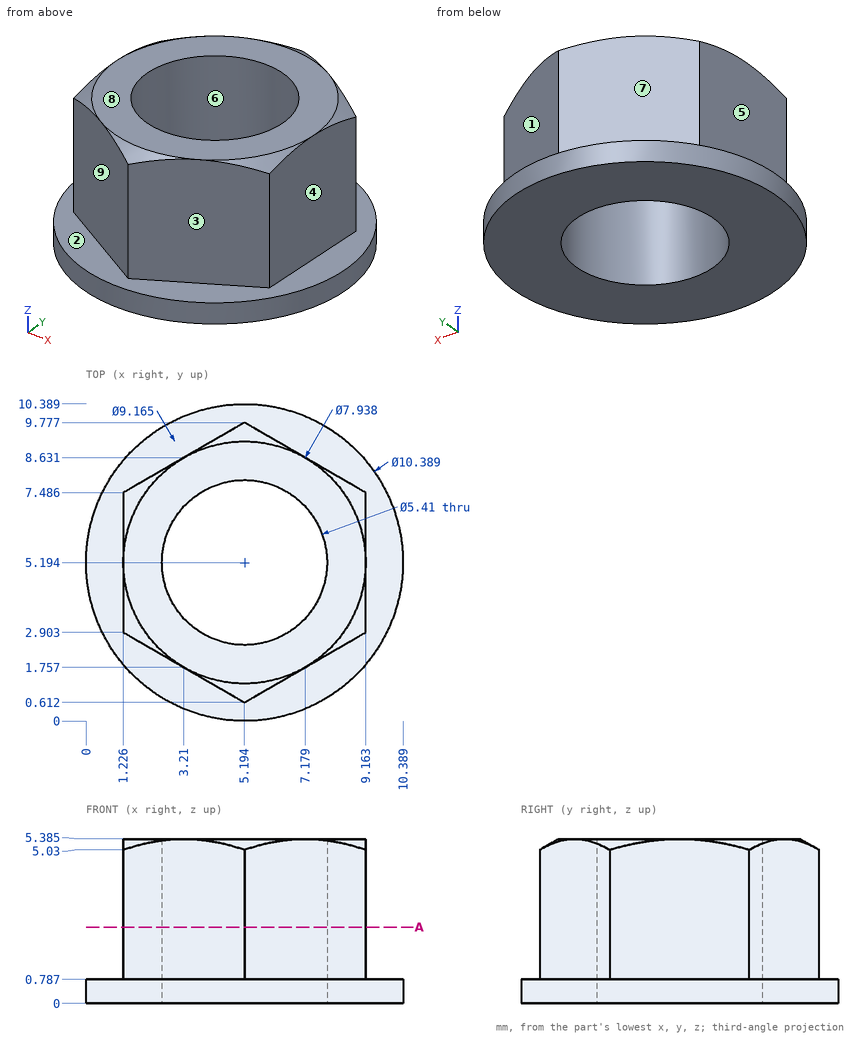
Drawing for the job (mm, zero at the part's lowest x, y, z). A direction names the side the tool comes from. Give positions to 0.01 mm unless a question says otherwise; leave off trailing zeros. Write each loop counter-clockwise with the first axis right and the second up, starting at its lowest first coordinate (ties: lowest second). Pieces come first, ordered by that corner, then holes. Notation, with made-up numbers: M 37.5,59.5 L 50.5,59.5 A29 cw 50.5,86.5 Z; hole C 31,88.5 d9. An arc over 180 degrees is marked long. Return JSON: item names as keys, results as strings. Group by question number.
(1) 3-axis set-ups, long thin cutter, end or side, ignore diameter. For the marked faces 1, 2, 3, 4 and 5: which of +Z, -Z, +X, -X, +Y, -Y reach the whole face in a straight line?
(2) Flat gauge pins, fed straight in: pin 1 Ø1.4 at (y, z) = (4.5, 3) entering from +X; pin 2 Ø2 at (x, z) = (3, 4) entering from +Y; pin 3 Ø2.5 at (y, z) = (6, 3.5) entering from -X. Where does each tip first touch, or does it go through?
(3) Mould opens along Y. For the marked faces 6, 7, 8 and 9 say: pulls with the +Y half, pulls with the -Y half, needs draft (parallel to the pull), parting line crosses it, or undercut.
(4) Drill centre lines: L1, parallel to Z at x = 10, y = 5; L2, parallel to X at y = 4.75, z = 0.35 (1 decimal); L3, parallel to X at y = 3.25, z = 4.7 (1 decimal). Where is each one in solid material? Low to high. Write a range as [from, to].
(5) Band-saw the part on A-A (z = 2.5). Give the cut face in (x, y) (1 decimal).
Entries:
{
 "1": {"face 1": "+Z, +X, +Y", "face 2": "+Z", "face 3": "+Z, +X, -Y", "face 4": "+Z, +X, +Y, -Y", "face 5": "+Z, -X, +Y, -Y"},
 "2": {"pin 1": "stops at x = 9.16", "pin 2": "stops at y = 9.09", "pin 3": "stops at x = 1.23"},
 "3": {"face 6": "undercut", "face 7": "pulls with the +Y half", "face 8": "needs draft", "face 9": "pulls with the -Y half"},
 "4": {"L1": "z = [0, 0.79]", "L2": "x = [0, 2.5], [7.9, 10.4]", "L3": "x = [1.2, 3.3], [7.1, 9.2]"},
 "5": {"outline": "M 1.2,2.9 L 5.2,0.6 L 9.2,2.9 L 9.2,7.5 L 5.2,9.8 L 1.2,7.5 Z; hole C 5.2,5.2 d5.4"}
}
